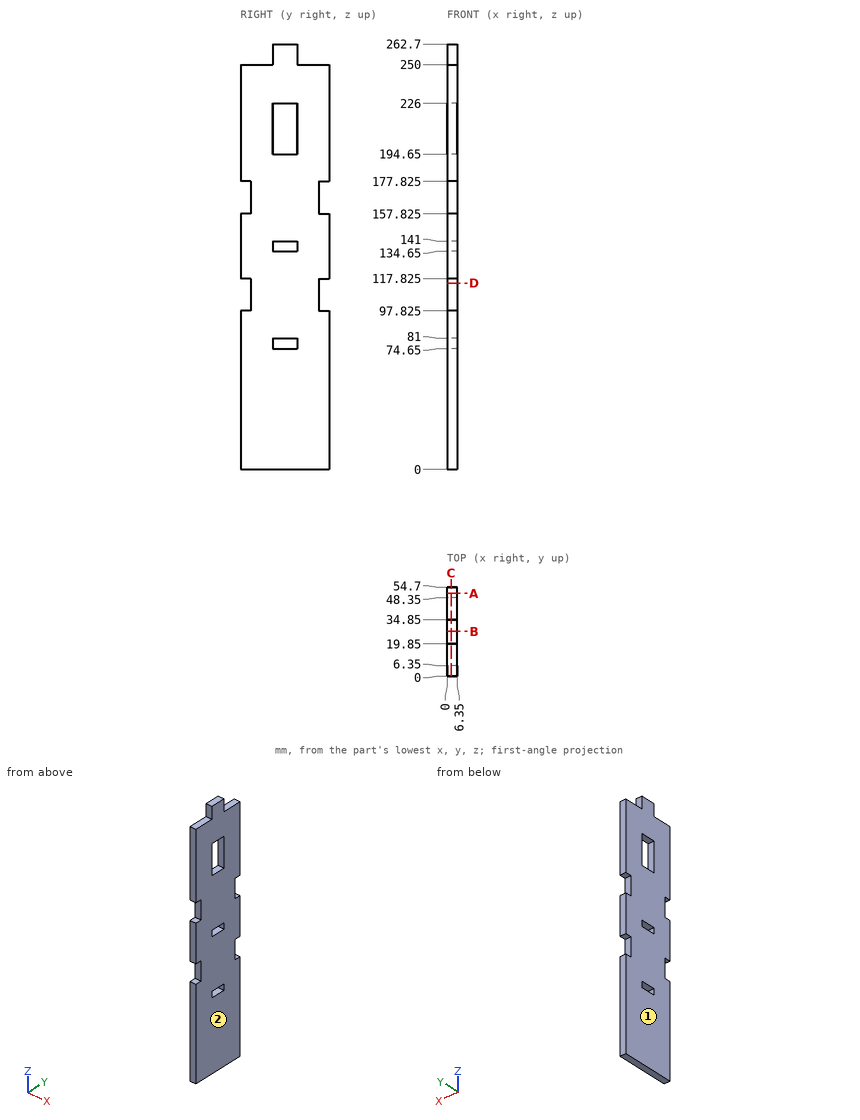
Could you check a few things on this drawing? It's one solid part, dimensions in mm from its lowest x, y, z. Coordinates: 2 decimals unless noted, no trailing zeros. Order: outer loops, then holes, each group sorted by start corner. A loop starts at its lowest first (then second) coordinate and runs counter-clockwise, first axis right, second up. Notation, with made-up numbers: M -6.5,73 L 17.5,73 A17 ccw 17.5,93 Z; hole C 29.25,82.25 d9. An arc over 180 degrees is marked long. Use one line per item in the form item = value. Start each with the question number.
1. We'd pull the mould along X, two halves only. Please class the marked faces 1 and 2: +X half, -X half, draft (parallel to the pull), parting line (faces both ways), or undercut.
2. Suppose I cut it at A-A on y = 51. Write out the boundary of the cut face in (x, z) (3 decimals).
3. Please list where these lines run through material, in increasing order: line 1 (Z direction, x = 4, y = 26.5); line 2 (Y direction, x = 5.5, z = 221); line 3 (Z direction, x = 2.5, y = 4.5) (3 decimals).
4. For pin 1 (1.9 mm diameter, centred on x = 2.5, y = 53, fed in from +Z); pin 2 (1.9 mm diameter, centred on x = 3.5, z = 106.5, fed in from +Y); pin 3 (3 mm diameter, centred on x = 4, z = 164, fed in from -Y), each with a flat end and sliding along its axis, tell me the tip position at first contact or that it passes through.
5. Suppose I cut it at D-D on z = 115. Write out the boundary of the cut face in (x, y).
6. Suppose I cut it at B-B on y = 27.5. Write out the boundary of the cut face in (x, z), then the cut area to 3 significant figures.
7. Suppose I cut it at C-C on x = 2.5. Count the separate pieces of the cut face and the enclosed holes in it, then the cut area to 3 significant figures.
Geometry says:
q1.face_1 = -X half
q1.face_2 = +X half
q2.outline = M 0,0 L 6.35,0 L 6.35,97.825 L 0,97.825 Z; M 0,117.825 L 6.35,117.825 L 6.35,157.825 L 0,157.825 Z; M 0,177.825 L 6.35,177.825 L 6.35,250 L 0,250 Z
q3.line_1 = 0 to 74.65, 81 to 134.65, 141 to 194.65, 226 to 262.7
q3.line_2 = 0 to 19.85, 34.85 to 54.7
q3.line_3 = 0 to 97.825, 117.825 to 157.825, 177.825 to 250
q4.pin_1 = 250
q4.pin_2 = 48.35
q4.pin_3 = 6.35
q5.outline = M 0,6.35 L 6.35,6.35 L 6.35,48.35 L 0,48.35 Z
q6.outline = M 0,0 L 6.35,0 L 6.35,74.65 L 0,74.65 Z; M 0,81 L 6.35,81 L 6.35,134.65 L 0,134.65 Z; M 0,141 L 6.35,141 L 6.35,194.65 L 0,194.65 Z; M 0,226 L 6.35,226 L 6.35,262.7 L 0,262.7 Z
q6.area = 1,390 mm^2
q7.separate_pieces = 1
q7.enclosed_holes = 3
q7.area = 12,700 mm^2
